from build123d import *

# Parameters (mm, degrees)
BOSS_EXTRUDE1_DEPTH       = 50.8
TAP_DRILL_FOR_8_32_TAP1_D = 3.4544
TAP_DRILL_FOR_8_32_TAP2_D = 3.4544


with BuildPart() as part:
    # Sketch1 → Boss-Extrude1 (new body)
    with BuildSketch(Plane.XY):
        Polygon((0, 0), (0, -30), (32, -30), (32, -28), (2, -28), (2, 0), align=None)
    extrude(amount=BOSS_EXTRUDE1_DEPTH)

    # Tap Drill for #8-32 Tap1 (through all)
    with Locations(Plane(origin=(0, -28, 0), x_dir=(1, 0, 0), z_dir=(0, 1, 0))):
        with Locations((19.05, -6.35), (19.05, -44.45), (19.05, -25.4)):
            Hole(TAP_DRILL_FOR_8_32_TAP1_D / 2)

    # Tap Drill for #8-32 Tap2 (through all)
    with Locations(Plane(origin=(2, 0, 0), x_dir=(0, 0, -1), z_dir=(1, 0, 0))):
        with Locations((-44.45, -12.7), (-6.35, -12.7), (-25.4, -12.7)):
            Hole(TAP_DRILL_FOR_8_32_TAP2_D / 2)


solid = part.part
The listing builds one solid part. Answer for the finished solid, in the listing's coordinates (mm). A direction names the side the tool comes from. Give positions to 0.01 mm unless a question says otherwise; leave off trailing zeros. Order: outer loops, then holes, each group sorted by start corner. A loop starts at its lowest first (then second) coordinate and runs counter-clockwise, first axis right, second up. Notation, with made-up numbers: (49.25, 62) - (85.25, 62) arc R25 cw to (85.25, 100) - close; hole circle Ø11 at (22, -7.5). An arc over 180 degrees is marked (long way). Use one line per item in the form item = value.
1) The mould has two halves that part along X. Classify faces 1 (the cylindrical face through (0.986, -13.362, 26.995)), 2 (the flat face through (2, -17, 25)), 3 (the cylindrical face through (20.32, -29.01, 24.23)): released by +X, released by -X, zero draft, split by the parting line, or undercut.
Verdict:
face_1 = zero draft
face_2 = released by +X
face_3 = undercut
2) Find section C-C on x = 19.05. Determine the outline of the cut face in (y, z).
Verdict:
outline = (-30, 0) - (-28, 0) - (-28, 4.62) - (-30, 4.62) - close; (-30, 8.08) - (-28, 8.08) - (-28, 23.67) - (-30, 23.67) - close; (-30, 27.13) - (-28, 27.13) - (-28, 42.72) - (-30, 42.72) - close; (-30, 46.18) - (-28, 46.18) - (-28, 50.8) - (-30, 50.8) - close
3) Each of these flat-tipped pins is pushed along its axis until it touches: pin 1 (8.5 mm diameter, centred on y = -18, z = 19.5, fed in from +X); pin 2 (4 mm diameter, centred on x = 19.05, z = 44.45, fed in from +Y). Where does it stop, or does it pass through?
Verdict:
pin_1 = 2
pin_2 = -28
4) Find section D-D on z = 15. Determine the outline of the cut face in (x, y).
Verdict:
outline = (0, -30) - (32, -30) - (32, -28) - (2, -28) - (2, 0) - (0, 0) - close
5) Find section A-A on z = 6.35. Determine the outline of the cut face in (x, y).
Verdict:
outline = (0, -30) - (17.32, -30) - (17.32, -28) - (2, -28) - (2, -14.43) - (0, -14.43) - close; (0, -10.97) - (2, -10.97) - (2, 0) - (0, 0) - close; (20.78, -30) - (32, -30) - (32, -28) - (20.78, -28) - close
6) Consider probe 1 along Z at (x, y) = (19.05, -28.85); probe 2 along X at (y, z) = (-28.6, 25.4); probe 3 along Y at (x, z) = (26.5, 15). Determine where each line is inside the solid, lowest interval first. Write a range as [from, to].
Verdict:
probe_1 = [0, 4.62], [8.08, 23.67], [27.13, 42.72], [46.18, 50.8]
probe_2 = [0, 17.32], [20.78, 32]
probe_3 = [-30, -28]
7) Find section B-B on y = -12.7. Determine the outline of the cut face in (x, z), and give its area (3 significant figures).
Verdict:
outline = (0, 0) - (2, 0) - (2, 4.62) - (0, 4.62) - close; (0, 8.08) - (2, 8.08) - (2, 23.67) - (0, 23.67) - close; (0, 27.13) - (2, 27.13) - (2, 42.72) - (0, 42.72) - close; (0, 46.18) - (2, 46.18) - (2, 50.8) - (0, 50.8) - close
area = 80.9 mm^2
8) For faces 4 (the flat face through (8.8, -28.3, 50.8)), 5 (the flat face through (17, -28, 25)), determine the directions among +Z, -Z, +X, -X, +Y, -Y from which every point of the face is accessible in a straight line to the end or side of a thin tool.
Verdict:
face_4 = +Z, +X, -X, +Y, -Y
face_5 = +Z, -Z, +X, +Y
